Read the model definition and answer for the solid it produces. Units are mm, in the model's axes. A direction names the side the tool comes from. Give positions to 0.01 mm unless a question says otherwise; leave off trailing zeros. Loops run counter-clockwise (first coordinate to the right, second up) from the corner with the lowest first, then second, coordinate; pieces in that order, holes last. Notation, with made-up numbers: (19, -21) -> (71, -21) arc R16 cw to (71, 9) -> close; hole circle Ø9 at (-25, 72.5). An arc over 180 degrees is marked (long way). Write each question's results on one line, items separated by ' | '. Start each with the question number.
Item 1: Each of these flat-tipped pins is pushed along its axis until it touches: P1, Ø0.6, axis at y = -0.5, z = 1, coming from the +X side; P2, Ø7.5, axis at x = 0.5, y = 0.5, coming from the -Z side; P3, Ø1.5, axis at x = -5, z = 0.5, coming from the -Y side. Where does it stop, or does it pass through?
Item 2: Determine the mould class of faces 4 (the flat face through (-3, -4, -2.9)), 5 (the flat face through (-2.5, 0, 1)), 6 (the cylindrical face through (4.57, 7.167, 0.986)) for opening direction Y: +Y half, -Y half, draft (parallel to the pull), parting line (faces both ways), or undercut.
Item 3: Find the intervals of material crossed by line 1 (X direction, y = 0, z = -1.4) (3 decimals); line 2 (Z direction, x = -5.5, y = -4.5), in increasing order.
Item 4: Section C-C on z = 1.6 is taken. Write down the section's boundary in (x, y), and give its area (3 significant figures).
Item 5: Which of the six approach directions +Z, -Z, +X, -X, +Y, -Y give full straight-line access (tool end or side, diameter ignored) to faces 1 (the flat face through (0, -2.5, 1)), 2 (the flat face through (4, 0, 2)), 3 (the cylindrical face through (-1.02, 4.59, -1.42))?
Item 6: Section D-D on x = -3.5 is taken. Write down the section's boundary in (y, z) (3 decimals), and give its area (3 significant figures).
Item 7: Section A-A on x = 0 is taken. Write down the section's boundary in (y, z) (3 decimals).
```python
from build123d import *

# Parameters (mm, degrees)
F0_R     = 8.5
F1_DEPTH = 2
F2_R     = 5.525
F3_DEPTH = 2.9
F4_R     = 4.7
F5_DEPTH = 3
F6_W     = 5
F6_H     = 5
F7_DEPTH = 25


with BuildPart() as f1:
    # F0 (on Top) → F1 (new body)
    with BuildSketch(Plane.XY):
        Circle(F0_R)
    extrude(amount=F1_DEPTH)

    # F2 (on face) → F3 (join)
    with BuildSketch(Plane(origin=(0, 0, 0), x_dir=(1, 0, 0), z_dir=(0, 0, -1))):
        Circle(F2_R)
    extrude(amount=F3_DEPTH)

    # F4 (on face) → F5 (cut)
    with BuildSketch(Plane(origin=(0, 0, -2.9), x_dir=(1, 0, 0), z_dir=(0, 0, -1))):
        Circle(F4_R)
    extrude(amount=-F5_DEPTH, mode=Mode.SUBTRACT)

    # F6 (on face) → F7 (cut)
    with BuildSketch(Plane.XY.offset(2)):
        Rectangle(F6_W, F6_H)
    extrude(amount=-F7_DEPTH, mode=Mode.SUBTRACT)


solid = f1.part
```
Findings:
1) P1: x = 8.5 | P2: z = 0.1 | P3: y = -7.36
2) face 4: draft | face 5: undercut | face 6: parting line
3) line 1: -5.525 to -4.7, 4.7 to 5.525 | line 2: 0 to 2
4) outline: circle Ø17 at (0, 0); hole (-2.5, -2.5) -> (2.5, -2.5) -> (2.5, 2.5) -> (-2.5, 2.5) -> close | area: 202 mm2
5) face 1: +Z, -Z | face 2: +Z, +X, -X, +Y, -Y | face 3: -Z
6) outline: (-7.746, 0) -> (-4.275, 0) -> (-4.275, -2.9) -> (-3.137, -2.9) -> (-3.137, 0.1) -> (3.137, 0.1) -> (3.137, -2.9) -> (4.275, -2.9) -> (4.275, 0) -> (7.746, 0) -> (7.746, 2) -> (-7.746, 2) -> close | area: 37.0 mm2
7) outline: (-8.5, 0) -> (-5.525, 0) -> (-5.525, -2.9) -> (-4.7, -2.9) -> (-4.7, 0.1) -> (-2.5, 0.1) -> (-2.5, 2) -> (-8.5, 2) -> close; (2.5, 0.1) -> (4.7, 0.1) -> (4.7, -2.9) -> (5.525, -2.9) -> (5.525, 0) -> (8.5, 0) -> (8.5, 2) -> (2.5, 2) -> close
